```python
from build123d import *

# Parameters (mm, degrees)
SKETCH_R        = 18
PAD_DEPTH       = 4
SKETCH002_R     = 26
SKETCH002_R_2   = 18
PAD001_DEPTH    = 5.4
SKETCH003_R     = 26
PAD002_DEPTH    = 4
SKETCH004_R     = 1.5
SKETCH004_R_2   = 7
POCKET_DEPTH    = 5
SKETCH005_R     = 1.5
POCKET001_DEPTH = 5
FILLET_R        = 6
SKETCH006_R     = 5
POCKET002_DEPTH = 15


with BuildPart() as part:
    # Sketch → Pad (new body)
    with BuildSketch(Plane.XY):
        with BuildLine():
            ThreePointArc((-39, 30), (-69, 0), (-39, -30))
            Line((-39, -30), (11, -30))
            ThreePointArc((11, -30), (41, 0), (11, 30))
            Line((-39, 30), (11, 30))
        make_face()
        Circle(SKETCH_R, mode=Mode.SUBTRACT)
    extrude(amount=PAD_DEPTH)

    # Sketch002 (on Face7 of Pad) → Pad001 (join)
    with BuildSketch(Plane.XY.offset(4)):
        Circle(SKETCH002_R)
        Circle(SKETCH002_R_2, mode=Mode.SUBTRACT)
    extrude(amount=PAD001_DEPTH)

    # Sketch003 (on Face10 of Pad001) → Pad002 (join)
    with BuildSketch(Plane.XY.offset(9.4)):
        Circle(SKETCH003_R)
    extrude(amount=PAD002_DEPTH)

    # Sketch004 (on Face12 of Pad002) → Pocket (cut)
    with BuildSketch(Plane.XY.offset(13.4)):
        with Locations((12.5, 0)):
            Circle(SKETCH004_R)
        with Locations((-12.5, 0)):
            Circle(SKETCH004_R)
        with Locations((0, 12.5)):
            Circle(SKETCH004_R)
        with Locations((0, -12.5)):
            Circle(SKETCH004_R)
        Circle(SKETCH004_R_2)
    extrude(amount=-POCKET_DEPTH, mode=Mode.SUBTRACT)

    # Sketch005 (on Face4 of Pocket) → Pocket001 (cut)
    with BuildSketch(Plane(origin=(0, 0, 0), x_dir=(1, 0, 0), z_dir=(0, 0, -1))):
        with Locations((-39, 27.5)):
            Circle(SKETCH005_R)
        with Locations((-14, 27.5)):
            Circle(SKETCH005_R)
        with Locations((11, 27.5)):
            Circle(SKETCH005_R)
        with Locations((30.445436, 19.445436)):
            Circle(SKETCH005_R)
        with Locations((38.5, 0)):
            Circle(SKETCH005_R)
        with Locations((30.445436, -19.445436)):
            Circle(SKETCH005_R)
        with Locations((11, -27.5)):
            Circle(SKETCH005_R)
        with Locations((-14, -27.5)):
            Circle(SKETCH005_R)
        with Locations((-39, -27.5)):
            Circle(SKETCH005_R)
        with Locations((-58.445436, -19.445436)):
            Circle(SKETCH005_R)
        with Locations((-66.5, 0)):
            Circle(SKETCH005_R)
        with Locations((-58.445436, 19.445436)):
            Circle(SKETCH005_R)
    extrude(amount=-POCKET001_DEPTH, mode=Mode.SUBTRACT)

    # Fillet
    fillet_edges = [part.edges().sort_by_distance(p)[0] for p in [
        (-26, 0, 13.4),
    ]]
    fillet(fillet_edges, radius=FILLET_R)

    # Sketch006 (on Face3 of Fillet) → Pocket002 (cut)
    with BuildSketch(Plane.XY.offset(4)):
        with Locations((-14, 27.5)):
            Circle(SKETCH006_R)
        with Locations((11, 27.5)):
            Circle(SKETCH006_R)
        with Locations((11, -27.5)):
            Circle(SKETCH006_R)
        with Locations((-14, -27.5)):
            Circle(SKETCH006_R)
    extrude(amount=POCKET002_DEPTH, mode=Mode.SUBTRACT)


solid = part.part
```
The listing builds one solid part. Answer for the finished solid, in the listing's coordinates (mm). A direction names the side the tool comes from. Round coordinates to 2 decimals unless told otherwise and drop trailing zeros. Loops run counter-clockwise (first coordinate to the right, second up) from the corner with the lowest first, then second, coordinate; pieces in that order, holes last. Notation, with made-up numbers: (-15, 78) - (-4, 78) arc R17 cw to (-4, 95) - close; hole circle Ø1 at (51, 85). An arc over 180 degrees is marked (long way). Use one line per item in the form item = value. Start each with the question number.
1. Given pin 1 Ø5 at (x, y) = (-14, -27.5) entering from +Z; pin 2 Ø1.8 at (x, y) = (-39, 27.5) entering from -Z; pin 3 Ø1 at (y, z) = (20, 8.5) entering from -X; pin 4 Ø5 at (x, z) = (17.5, 8.5) entering from +Y, each flat-ended and moving along its own axis, determine where each tip first touches the part or whether it passes through.
2. A tool of negligible diameter and unlimited length cuts with its end or side. For faces 4 (the face through (-11.72, -23.05, 6.32)), 5 (the face through (-2.343, 17.847, 4.634)), 6 (the face through (-2.37, -25.89, 5.68)), from which of +Z, -Z, +X, -X, +Y, -Y can it reach the whole face along a straight path? Write none if from no direction.
3. Consider line 1 (X direction, y = -27.5, z = 2.3); line 2 (Y direction, x = -14, z = 2.55); line 3 (Y direction, x = -39, z = 2.4). Determine where each line is inside the solid, lowest interval first. Write a range as [from, to].
4. The part is cut by section A-A on y = 0. Give the number of separate pieces and of enclosed holes in the cut face, then the cut area to 3 significant figures.
5. For a pull along Y with two mould halves and no side action, classify faces 1 (the face through (40.993, -0.66, 1.972)), 2 (the face through (9.19, -22.84, 7.57)), 3 (the face through (-14, -29, 2)) as pulls with the +Y half, pulls with the -Y half, needs draft (parallel to the pull), parting line crosses it, or undercut.
6. The part is cut by section C-C on z = 5.75. Determine the outline of the cut face in (x, y).
7. The part is cut by section B-B on x = 0. Determine the outline of the cut face in (y, z).
8. The part is cut by section D-D on y = -27.5. Determine the outline of the cut face in (x, z).
Geometry check:
q1.pin_1 = 4
q1.pin_2 = through
q1.pin_3 = -17.06
q1.pin_4 = 21.16
q2.face_4 = +Z, -X, -Y
q2.face_5 = -Z
q2.face_6 = +Z, -Y
q3.line_1 = [-50.99, -40.5], [-37.5, -15.5], [-12.5, 9.5], [12.5, 22.99]
q3.line_2 = [-30, -29], [-26, -11.31], [11.31, 26], [29, 30]
q3.line_3 = [-30, -29], [-26, 26], [29, 30]
q4.separate_pieces = 6
q4.enclosed_holes = 0
q4.area = 471 mm^2
q5.face_1 = parting line crosses it
q5.face_2 = pulls with the -Y half
q5.face_3 = undercut
q6.outline = (-12.75, -22.66) arc R5 cw to (-10.82, -23.64) arc R26 ccw to (6.59, -25.15) arc R5 cw to (12.58, -22.76) arc R26 ccw to (12.58, 22.76) arc R5 cw to (6.59, 25.15) arc R26 ccw to (-10.82, 23.64) arc R5 cw to (-12.75, 22.66) arc R26 ccw to start; hole circle Ø36 at (0, 0)
q7.outline = (-30, 0) - (-18, 0) - (-18, 9.4) - (-14, 9.4) - (-14, 13.4) - (-20, 13.4) arc R6 ccw to (-26, 7.4) - (-26, 4) - (-30, 4) - close; (-11, 9.4) - (-7, 9.4) - (-7, 13.4) - (-11, 13.4) - close; (7, 9.4) - (11, 9.4) - (11, 13.4) - (7, 13.4) - close; (14, 9.4) - (18, 9.4) - (18, 0) - (30, 0) - (30, 4) - (26, 4) - (26, 7.4) arc R6 ccw to (20, 13.4) - (14, 13.4) - close
q8.outline = (-50.99, 0) - (-40.5, 0) - (-40.5, 4) - (-50.99, 4) - close; (-37.5, 0) - (-15.5, 0) - (-15.5, 4) - (-37.5, 4) - close; (-12.5, 0) - (9.5, 0) - (9.5, 4) - (-12.5, 4) - close; (12.5, 0) - (22.99, 0) - (22.99, 4) - (12.5, 4) - close
